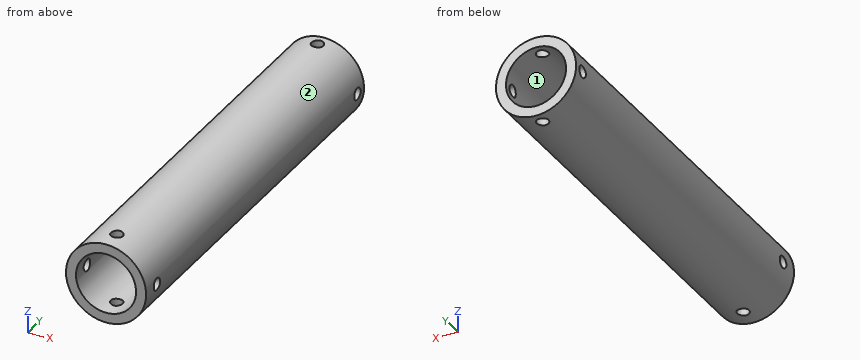
```python
from build123d import *

# Parameters (mm, degrees)
SKETCH1_R         = 12.7
SKETCH1_R_2       = 9.525
ELTUBO_DEPTH      = 127
SETSCREW_REACH    = 132.136
SETSCREW_BORE_R   = 1.89865
CIRPATTERN1_COUNT = 4


with BuildPart() as part:
    # Sketch1 → ElTubo (new body)
    with BuildSketch(Plane(origin=(0, 0, 0), x_dir=(1, 0, 0), z_dir=(0, 1, 0))):
        with Locations(Location((0, 0, 0), (0, 0, 270))):
            Circle(SKETCH1_R)
        with Locations(Location((0, 0, 0), (0, 0, 270))):
            Circle(SKETCH1_R_2, mode=Mode.SUBTRACT)
    extrude(amount=ELTUBO_DEPTH)

    # SetScrew bore → SetScrew (cut, up to next)
    with BuildSketch(Plane.ZY.offset(12.7), mode=Mode.PRIVATE) as setscrew_sk1:
        with Locations((0, 6.35)):
            Circle(SETSCREW_BORE_R)
    setscrew_tool1 = extrude(setscrew_sk1.sketch, amount=-SETSCREW_REACH, mode=Mode.PRIVATE) & part.part
    # SetScrew bore → SetScrew (cut, up to next)
    with BuildSketch(Plane.ZY.offset(12.7), mode=Mode.PRIVATE) as setscrew_sk2:
        with Locations((0, 123.19)):
            Circle(SETSCREW_BORE_R)
    setscrew_tool2 = extrude(setscrew_sk2.sketch, amount=-SETSCREW_REACH, mode=Mode.PRIVATE) & part.part
    setscrew_1 = setscrew_tool1.solids().sort_by_distance((-12.7, 6.35, 0))[0]
    add(setscrew_1, mode=Mode.SUBTRACT)
    setscrew_2 = setscrew_tool2.solids().sort_by_distance((-12.7, 123.19, 0))[0]
    add(setscrew_2, mode=Mode.SUBTRACT)
    setscrew = setscrew_1 + setscrew_2  # SetScrew as one shape, for the pattern or mirror that repeats it

    # CirPattern1: SetScrew ×4 about axis
    cirpattern1_axis = Axis((0, 127, 0), (0, -1, 0))
    for i in range(1, CIRPATTERN1_COUNT):
        add(setscrew.rotate(cirpattern1_axis, i * 360 / CIRPATTERN1_COUNT), mode=Mode.SUBTRACT)


solid = part.part
```
Geometry check sheet. Reference: the model listing, model coordinates, mm. Face numbers are marked on the shaded views. Round coordinates to 2 decimals unless told otherwise and drop trailing zeros. Loops run counter-clockwise (first coordinate to the right, second up) from the corner with the lowest first, then second, coordinate; pieces in that order, holes last. Notation, with made-up numbers: (3, -14) - (48, -14) arc R27 ccw to (48, 16) - close; hole circle Ø1 at (73, -3). An arc over 180 degrees is marked (long way). Use a Markdown table: item, result.
Q1. Material ranges on line 1 (X direction, y = 33.5, z = 0) (3 decimals); line 2 (Z direction, x = 3.5, y = 42); line 3 (Z direction, x = 2.25, y = 62.5), recorded low to high.
Solutions:
| item | result |
|---|---|
| line 1 | x = -12.7 to -9.525, 9.525 to 12.7 |
| line 2 | z = -12.21 to -8.86, 8.86 to 12.21 |
| line 3 | z = -12.5 to -9.26, 9.26 to 12.5 |
Q2. Go/stop test with flat-tipped pins: P1, Ø8, axis at y = 32, z = -6.5, coming from the -X side; P2, Ø10, axis at y = 39.5, z = -3.5, coming from the -X side; P3, Ø3, axis at y = 123.19, z = 0, coming from the +X side; P4, Ø3, axis at y = 20, z = 8, coming from the -X side. Record where each tip stops, or that it passes through.
Solutions:
| item | result |
|---|---|
| P1 | stops at x = -12.45 |
| P2 | stops at x = -12.7 |
| P3 | passes through |
| P4 | stops at x = -10.91 |
Q3. Cross-section at D-D on z = -7. Record the cut outline in (x, y).
Solutions:
| item | result |
|---|---|
| outline | (-10.6, 0) - (-6.46, 0) - (-6.46, 127) - (-10.6, 127) - close; (6.46, 0) - (10.6, 0) - (10.6, 127) - (6.46, 127) - close |
Q4. Cross-section at A-A on z = 0. Record the cut outline in (x, y) (3 decimals).
Solutions:
| item | result |
|---|---|
| outline | (-12.7, 0) - (-9.525, 0) - (-9.525, 4.451) - (-12.7, 4.451) - close; (-12.7, 8.249) - (-9.525, 8.249) - (-9.525, 121.291) - (-12.7, 121.291) - close; (-12.7, 125.089) - (-9.525, 125.089) - (-9.525, 127) - (-12.7, 127) - close; (9.525, 0) - (12.7, 0) - (12.7, 4.451) - (9.525, 4.451) - close; (9.525, 8.249) - (12.7, 8.249) - (12.7, 121.291) - (9.525, 121.291) - close; (9.525, 125.089) - (12.7, 125.089) - (12.7, 127) - (9.525, 127) - close |
Q5. Cross-section at B-B on x = 0. Record the cut outline in (y, z) (3 decimals).
Solutions:
| item | result |
|---|---|
| outline | (0, -12.7) - (4.451, -12.7) - (4.451, -9.525) - (0, -9.525) - close; (0, 9.525) - (4.451, 9.525) - (4.451, 12.7) - (0, 12.7) - close; (8.249, -12.7) - (121.291, -12.7) - (121.291, -9.525) - (8.249, -9.525) - close; (8.249, 9.525) - (121.291, 9.525) - (121.291, 12.7) - (8.249, 12.7) - close; (125.089, -12.7) - (127, -12.7) - (127, -9.525) - (125.089, -9.525) - close; (125.089, 9.525) - (127, 9.525) - (127, 12.7) - (125.089, 12.7) - close |
Q6. Cross-section at C-C on y = 6.35. Record the cut outline in (x, z) (3 decimals), plus the area to 3 significant figures.
Solutions:
| item | result |
|---|---|
| outline | (-12.557, -1.899) arc R12.7 ccw to (-1.899, -12.557) - (-1.899, -9.334) arc R9.525 cw to (-9.334, -1.899) - close; (-12.557, 1.899) - (-9.334, 1.899) arc R9.525 cw to (-1.899, 9.334) - (-1.899, 12.557) arc R12.7 ccw to start; (1.899, -12.557) arc R12.7 ccw to (12.557, -1.899) - (9.334, -1.899) arc R9.525 cw to (1.899, -9.334) - close; (1.899, 9.334) arc R9.525 cw to (9.334, 1.899) - (12.557, 1.899) arc R12.7 ccw to (1.899, 12.557) - close |
| area | 173 mm2 |
Q7. Draft check along Z on the marked faces 1 and 2. Enter one of: released by +Z, released by -Z, zero draft, split by the parting line, or undercut.
Solutions:
| item | result |
|---|---|
| face 1 | undercut |
| face 2 | split by the parting line |
